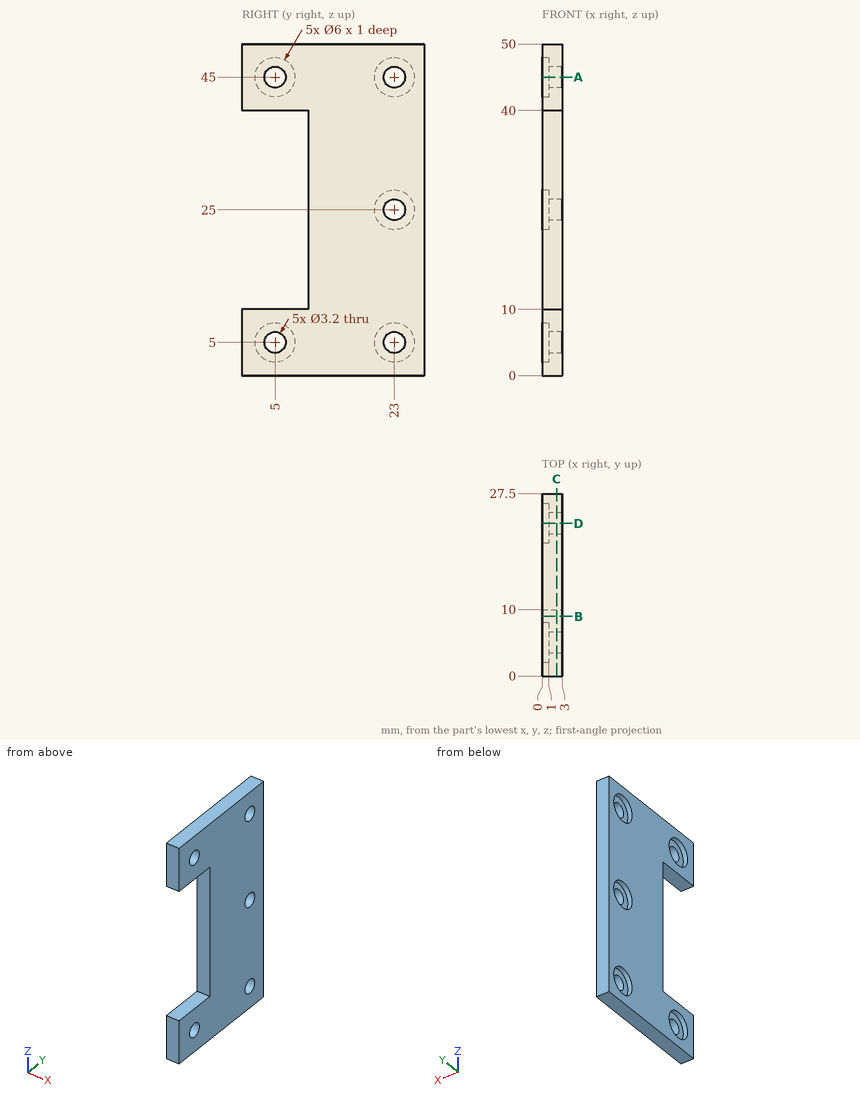
Verification items for this drawing (mm, ordinates from the low corner). Coordinates: 2 decimals unless noted, no trailing zeros. Write each loop counter-clockwise with the first axis right and the second up, starting at its lowest first coordinate (ties: lowest second). Pieces come first, ordered by that corner, then holes. Notation, with made-up numbers: (-35.75, -5) -> (12.25, -5) arc R20 ccw to (12.25, 18) -> close; hole circle Ø5 at (-7.75, 65.25). An arc over 180 degrees is marked (long way). One line per item, written item: value. Start each with the question number.
Q1. Cross-section at A-A on z = 45. Enter the section's corners in (x, y), and give its area (3 significant figures).
Q2. Cross-section at B-B on y = 9. Enter the section's corners in (x, z).
Q3. Cross-section at D-D on y = 23. Enter the section's corners in (x, z).
Q4. Thickness scan on L1, parallel to Z at x = 1.7, y = 5; L2, parallel to Y at x = 0.7, z = 5; L3, parallel to Z at x = 2.2, y = 23. Record the ranges inside material, lowest first. Write a range as from..to.
Q5. Cross-section at C-C on x = 2.15. Enter the section's corners in (y, z), and give its area (3 significant figures).
Q6. Go/stop test with flat-tipped pins: P1, Ø3.5, axis at y = 5, z = 5, coming from the -X side; P2, Ø9.5, axis at y = 23, z = 45, coming from the +X side. Record where each tip stops, or that it passes through.
Checked values:
1. outline: (0, 0) -> (3, 0) -> (3, 3.4) -> (1, 3.4) -> (1, 2) -> (0, 2) -> close; (0, 8) -> (1, 8) -> (1, 6.6) -> (3, 6.6) -> (3, 21.4) -> (1, 21.4) -> (1, 20) -> (0, 20) -> close; (0, 26) -> (1, 26) -> (1, 24.6) -> (3, 24.6) -> (3, 27.5) -> (0, 27.5) -> close
1. area: 57.7 mm²
2. outline: (0, 0) -> (3, 0) -> (3, 10) -> (0, 10) -> close; (0, 40) -> (3, 40) -> (3, 50) -> (0, 50) -> close
3. outline: (0, 0) -> (3, 0) -> (3, 3.4) -> (1, 3.4) -> (1, 2) -> (0, 2) -> close; (0, 8) -> (1, 8) -> (1, 6.6) -> (3, 6.6) -> (3, 23.4) -> (1, 23.4) -> (1, 22) -> (0, 22) -> close; (0, 28) -> (1, 28) -> (1, 26.6) -> (3, 26.6) -> (3, 43.4) -> (1, 43.4) -> (1, 42) -> (0, 42) -> close; (0, 48) -> (1, 48) -> (1, 46.6) -> (3, 46.6) -> (3, 50) -> (0, 50) -> close
4. L1: z = 0..3.4, 6.6..10, 40..43.4, 46.6..50
4. L2: y = 0..2, 8..20, 26..27.5
4. L3: z = 0..3.4, 6.6..23.4, 26.6..43.4, 46.6..50
5. outline: (0, 0) -> (27.5, 0) -> (27.5, 50) -> (0, 50) -> (0, 40) -> (10, 40) -> (10, 10) -> (0, 10) -> close; hole circle Ø3.2 at (5, 5); hole circle Ø3.2 at (5, 45); hole circle Ø3.2 at (23, 5); hole circle Ø3.2 at (23, 25); hole circle Ø3.2 at (23, 45)
5. area: 1,030 mm²
6. P1: stops at x = 1
6. P2: stops at x = 3
